Design review of the part built by this model. Coordinates are the model's own, in mm. A direction names the side the tool comes from. Coordinates: 2 decimals unless noted, no trailing zeros. Write each loop counter-clockwise with the first axis right and the second up, starting at its lowest first coordinate (ties: lowest second). Pieces come first, ordered by that corner, then holes.
Q1. For probe 1 along X at (y, z) = (-3, 1.5); probe 2 along Y at (x, z) = (2, -2.75); probe 3 along Y at (x, z) = (-1.75, 2), list the stretches that pass through material, from the lowest coordinate up.
Q2. Machinability: for faces 1 (the flat face through (-1.5, 1, 0)), 2 (the flat face through (0, 8.5, 0)), 3 (the flat face through (1.5, 1, 0)), which of the approach directions +Z, -Z, +X, -X, +Y, -Y give a long, thin tool a straight path to every point of the face, cutting with its end or side? Answer none if there is none.
Q3. Take a section at A-A (z = 3.25). Give the boundary of the cut face in (x, y), and give its area (3 significant figures).
Q4. Take a section at C-C (x = -2.5). Give the boundary of the cut face in (y, z).
Q5. Take a section at B-B (y = 5.5). Give the boundary of the cut face in (x, z).
Q6. Insertion check: pin 1 (1 mm diameter, centred on y = -4, z = -2, fed in from -X). The pin has a flat end and moves straight along its axis. Give the tip position at first contact, or say it passes through.
```python
from build123d import *

# Parameters (mm, degrees)
SKETCH1_W           = 3
SKETCH1_H           = 13
BOSS_EXTRUDE1_DEPTH = 4
BOSS_EXTRUDE2_DEPTH = 8
CHAMFER1_SIZE       = 1
CHAMFER1_SIZE2      = 1.732050808


with BuildPart() as part:
    # Sketch1 → Boss-Extrude1 (new, symmetric)
    with BuildSketch(Plane.XY):
        Rectangle(SKETCH1_W, SKETCH1_H)
    extrude(amount=BOSS_EXTRUDE1_DEPTH, both=True)

    # Sketch2 → Boss-Extrude2 (add)
    with BuildSketch(Plane.XY.offset(4)):
        Polygon((-1.5, 6.5), (-3.5, 8.5), (3.5, 8.5), (1.5, 6.5), align=None)
    extrude(amount=-BOSS_EXTRUDE2_DEPTH)

    # Chamfer1
    chamfer1_edges = [part.edges().sort_by_distance(p)[0] for p in [
        (1.5, -6.5, 0),
        (-1.5, -6.5, 0),
    ]]
    chamfer1_side = [part.faces().sort_by_distance(p)[0] for p in [
        (0, -6.5, 0),
    ]]
    chamfer(chamfer1_edges, length=CHAMFER1_SIZE, length2=CHAMFER1_SIZE2, reference=chamfer1_side[0])


solid = part.part
```
Response:
1. probe 1: x = -1.5 to 1.5
1. probe 2: y = 7 to 8.5
1. probe 3: y = 6.75 to 8.5
2. face 1: +Z, -Z, -X, -Y
2. face 2: +Z, -Z, +X, -X, +Y
2. face 3: +Z, -Z, +X, -Y
3. outline: (-3.5, 8.5) - (-1.5, 6.5) - (-1.5, -4.77) - (-0.5, -6.5) - (0.5, -6.5) - (1.5, -4.77) - (1.5, 6.5) - (3.5, 8.5) - close
3. area: 47.3 mm2
4. outline: (7.5, -4) - (8.5, -4) - (8.5, 4) - (7.5, 4) - close
5. outline: (-1.5, -4) - (1.5, -4) - (1.5, 4) - (-1.5, 4) - close
6. pin 1: stops at x = -1.5
